```python
from build123d import *

# Parameters (mm, degrees)
BOSS_EXTRUDE1_DEPTH = 10
BOSS_EXTRUDE3_DEPTH = 50
CUT_EXTRUDE2_START  = -10
CUT_EXTRUDE2_DEPTH  = 10
CUT_EXTRUDE3_START  = -10
CUT_EXTRUDE3_DEPTH  = 10
SKETCH9_R           = 11
CUT_EXTRUDE4_DEPTH  = 10
SKETCH10_R          = 11
CUT_EXTRUDE5_DEPTH  = 10


# Read off the part's stored shape, not the designer's step: Cut-Extrude2, Cut-Extrude3
with BuildPart() as part:
    # Sketch2 → Boss-Extrude1 (new body)
    with BuildSketch(Plane(origin=(0, 0, 0), x_dir=(1, 0, 0), z_dir=(0, 1, 0))):
        with BuildLine():
            ThreePointArc((0, 20), (-12.427112426, 15.670573594), (-19.473997983, 4.556687675))
            Line((-19.473997983, 4.556687675), (-26.455560952, -25.280543414))
            Line((-26.455560952, -25.280543414), (-15.63841821, -29.017513463))
            Line((-15.63841821, -29.017513463), (-18.903729183, -38.469378055))
            Line((-18.903729183, -38.469378055), (0, -45))
            Line((0, -45), (0, -12.5))
            ThreePointArc((0, -12.5), (-12.5, 0), (0, 12.5))
            Line((0, 12.5), (0, 20))
        make_face()
        with BuildLine():
            ThreePointArc((19.473997983, 4.556687675), (12.427112426, 15.670573594), (0, 20))
            Line((0, 20), (0, 12.5))
            ThreePointArc((0, 12.5), (8.838834765, 8.838834765), (12.5, 0))
            ThreePointArc((12.5, 0), (8.838834765, -8.838834765), (0, -12.5))
            Line((0, -12.5), (0, -45))
            Line((0, -45), (18.903729183, -38.469378055))
            Line((18.903729183, -38.469378055), (15.63841821, -29.017513463))
            Line((15.63841821, -29.017513463), (26.455560952, -25.280543414))
            Line((26.455560952, -25.280543414), (19.473997983, 4.556687675))
        make_face()
        Polygon((44.52777222, -19.037183791), (26.455560952, -25.280543414), (15.63841821, -29.017513463), (18.903729183, -38.469378055), (47.793083193, -28.489048382), align=None)
        Polygon((-15.63841821, -29.017513463), (-26.455560952, -25.280543414), (-44.52777222, -19.037183791), (-47.793083193, -28.489048382), (-18.903729183, -38.469378055), align=None)
    extrude(amount=BOSS_EXTRUDE1_DEPTH)

    # Sketch6 → Boss-Extrude3 (add)
    with BuildSketch(Plane(origin=(0, 10, 0), x_dir=(1, 0, 0), z_dir=(0, 1, 0))):
        Polygon((47.793083193, -28.489048382), (44.52777222, -19.037183791), (15.63841821, -29.017513463), (18.903729183, -38.469378055), align=None)
        Polygon((-47.793083193, -28.489048382), (-44.52777222, -19.037183791), (-15.63841821, -29.017513463), (-18.903729183, -38.469378055), align=None)
    extrude(amount=BOSS_EXTRUDE3_DEPTH)

    # Cut-Extrude2 outline → Cut-Extrude2 (cut)
    with BuildSketch(Plane(origin=(-13.888474723, 0, 40.201984913), x_dir=(0.9451864591285483, 0, 0.32653109726339585), z_dir=(-0.3265310972633958, 0, 0.9451864591285482)).offset(CUT_EXTRUDE2_START)):
        with BuildLine():
            ThreePointArc((-35.870814845, 44.066794658), (-20.588457734, 58.63224641), (-5.306100623, 44.066794658))
            Line((-5.306100623, 44.066794658), (-5.306100623, 60))
            Line((-5.306100623, 60), (-35.870814845, 60))
            Line((-35.870814845, 60), (-35.870814845, 44.066794658))
        make_face()
    extrude(amount=CUT_EXTRUDE2_DEPTH, mode=Mode.SUBTRACT)

    # Cut-Extrude3 outline → Cut-Extrude3 (cut)
    with BuildSketch(Plane(origin=(13.888474723, 0, 40.201984913), x_dir=(0.9451864591285483, 0, -0.3265310972633959), z_dir=(0.3265310972633959, 0, 0.9451864591285483)).offset(CUT_EXTRUDE3_START)):
        with BuildLine():
            ThreePointArc((5.306100623, 43.936741919), (20.588457734, 58.743356846), (35.870814845, 43.936741919))
            Line((35.870814845, 43.936741919), (35.870814845, 60))
            Line((35.870814845, 60), (5.306100623, 60))
            Line((5.306100623, 60), (5.306100623, 43.936741919))
        make_face()
    extrude(amount=CUT_EXTRUDE3_DEPTH, mode=Mode.SUBTRACT)

    # Sketch9 → Cut-Extrude4 (cut)
    with BuildSketch(Plane(origin=(-13.888474723, 0, 40.201984913), x_dir=(0.9451864591285483, 0, 0.32653109726339585), z_dir=(-0.3265310972633958, 0, 0.9451864591285482))):
        with Locations((-20.588457734, 43.33224641)):
            Circle(SKETCH9_R)
    extrude(amount=-CUT_EXTRUDE4_DEPTH, mode=Mode.SUBTRACT)

    # Sketch10 → Cut-Extrude5 (cut)
    with BuildSketch(Plane(origin=(13.888474723, 0, 40.201984913), x_dir=(0.9451864591285483, 0, -0.3265310972633959), z_dir=(0.3265310972633959, 0, 0.9451864591285483))):
        with Locations((20.588457734, 43.453356846)):
            Circle(SKETCH10_R)
    extrude(amount=-CUT_EXTRUDE5_DEPTH, mode=Mode.SUBTRACT)


solid = part.part
```
Can you work these out from the model? Positions are in its coordinate system, mm. A direction names the side the tool comes from. Round coordinates to 2 decimals unless told otherwise and drop trailing zeros. Order: outer loops, then holes, each group sorted by start corner. A loop starts at its lowest first (then second) coordinate and runs counter-clockwise, first axis right, second up.
(1) If we section it at B-B (z = 3): Please give me the cut outline in (x, y), plus the area to 3 significant figures.
Results are:
outline: (-21.24, 0) - (-12.13, 0) - (-12.13, 10) - (-21.24, 10) - close; (12.13, 0) - (21.24, 0) - (21.24, 10) - (12.13, 10) - close
area: 182 mm2
(2) On a 3-axis mill with a long thin cutter (end or side, diameter ignored), from which of +Z, -Z, +X, -X, +Y, -Y can I reach the whole of each face in a straight line? I mean faces 4 (the face through (-17.25, 26.79, 33.68)), 5 (the face through (-22.916, 4.93, 10.153)), 6 (the face through (-32, 58.63, 28.58)). Say none if no direction works.
Results are:
face 4: +Z, +Y
face 5: -Z, +Y, -Y
face 6: +Y
(3) I'm going to push flat-ended pins straight in: pin 1 (4 mm diameter, centred on x = -17, z = 6.5, fed in from +Y); pin 2 (6 mm diameter, centred on x = 22.5, y = 15, fed in from +Z); pin 3 (6 mm diameter, centred on x = -36, y = 17.5, fed in from -Z). Where does each tip first touch, or does it pass through?
Results are:
pin 1: stops at y = 10
pin 2: stops at z = 38.26
pin 3: stops at z = 20.95
(4) We'd pull the mould along X, two halves only. Please class faces 1 (the face through (-1, 0, 19)), 2 (the face through (23.014, 4.93, 10.571)), 3 (the face through (-46.14, 21.72, 23.7)): +X half, -X half, draft (parallel to the pull), parting line (faces both ways), or undercut.
Results are:
face 1: draft
face 2: undercut
face 3: -X half
(5) If I drill on L1, parallel to Y at x = -3.5, z = 39; L2, parallel to Y at x = 38, z = 26; L3, parallel to Y at x = 34.5, z = 27, over which ranges is the centre line in solid material (lowest first)?
Results are:
L1: y = 0 to 10
L2: y = 0 to 34.84, 52.07 to 57.13
L3: y = 0 to 32.93, 53.98 to 58.4
(6) If we section it at A-A (y = 17.5): Please give me the cut outline in (x, z).
Results are:
outline: (-47.79, 28.49) - (-44.53, 19.04) - (-15.64, 29.02) - (-18.9, 38.47) - close; (15.64, 29.02) - (44.53, 19.04) - (47.79, 28.49) - (18.9, 38.47) - close
